```python
from build123d import *

# Parameters (mm, degrees)
SKETCH1_W           = 27.94
SKETCH1_H           = 17.78
SKETCH1_W_2         = 2.54
SKETCH1_H_2         = 12.7
BOSS_EXTRUDE2_DEPTH = 2.54
SKETCH3_R           = 1.27
BOSS_EXTRUDE3_DEPTH = 3.302
SKETCH6_W           = 2.503557337
SKETCH6_H           = 12.554229347
BOSS_EXTRUDE6_DEPTH = 3.302
SKETCH4_W           = 27.94
SKETCH4_H           = 17.78
SKETCH4_W_2         = 2.54
SKETCH4_H_2         = 12.7
BOSS_EXTRUDE7_DEPTH = 2.54


with BuildPart() as part:
    # Sketch1 → Boss-Extrude2 (new body)
    with BuildSketch(Plane(origin=(0, 0, 0), x_dir=(1, 0, 0), z_dir=(0, 1, 0))):
        Rectangle(SKETCH1_W, SKETCH1_H)
        with Locations((-10.20489899, 0)):
            Rectangle(SKETCH1_W_2, SKETCH1_H_2, mode=Mode.SUBTRACT)
        with Locations((10.20489899, 0)):
            Rectangle(SKETCH1_W_2, SKETCH1_H_2, mode=Mode.SUBTRACT)
    extrude(amount=BOSS_EXTRUDE2_DEPTH)

    # Sketch3 → Boss-Extrude3 (add)
    with BuildSketch(Plane(origin=(0, 2.54, 0), x_dir=(1, 0, 0), z_dir=(0, 1, 0))):
        with Locations(Location((-5.318941048, 2.54, 0), (0, 0, 90))):
            Circle(SKETCH3_R)
        with Locations(Location((5.318941048, 2.54, 0), (0, 0, 90))):
            Circle(SKETCH3_R)
    extrude(amount=BOSS_EXTRUDE3_DEPTH)

    # Sketch6 → Boss-Extrude6 (add)
    with BuildSketch(Plane(origin=(0, 2.54, 0), x_dir=(1, 0, 0), z_dir=(0, 1, 0))):
        Polygon((-7.215647318, 4.760339872), (7.384221332, 4.760339872), (7.384221332, -8.817114674), (13.988221332, -8.817114674), (13.97, 8.89), (-13.97, 8.89), (-13.97, -8.89), (-7.347778668, -8.89), align=None)
        with Locations((10.223120322, 0.072885327)):
            Rectangle(SKETCH6_W, SKETCH6_H, mode=Mode.SUBTRACT)
        with Locations((-10.186677659, 0.072885327)):
            Rectangle(SKETCH6_W, SKETCH6_H, mode=Mode.SUBTRACT)
    extrude(amount=BOSS_EXTRUDE6_DEPTH)

    # Sketch4 → Boss-Extrude7 (add)
    with BuildSketch(Plane(origin=(0, 5.842, 0), x_dir=(1, 0, 0), z_dir=(0, 1, 0))):
        with Locations((0.018221332, 0.072885326)):
            Rectangle(SKETCH4_W, SKETCH4_H)
        with Locations((-10.186677658, 0.072885326)):
            Rectangle(SKETCH4_W_2, SKETCH4_H_2, mode=Mode.SUBTRACT)
        with Locations((10.223120322, 0.072885326)):
            Rectangle(SKETCH4_W_2, SKETCH4_H_2, mode=Mode.SUBTRACT)
    extrude(amount=BOSS_EXTRUDE7_DEPTH)


solid = part.part
```
Geometry: final body of the model. Coordinates: model frame, mm. A direction names the side the tool comes from. Round coordinates to 2 decimals unless told otherwise and drop trailing zeros. Loops run counter-clockwise (first coordinate to the right, second up) from the corner with the lowest first, then second, coordinate; pieces in that order, holes last.
Item 1: Section D-D, the plane y = 1.25. Output: boundary loops of the cut face in (x, z).
Checked values:
outline: (-13.97, -8.89) - (13.97, -8.89) - (13.97, 8.89) - (-13.97, 8.89) - close; hole (-11.47, -6.35) - (-8.93, -6.35) - (-8.93, 6.35) - (-11.47, 6.35) - close; hole (8.93, -6.35) - (11.47, -6.35) - (11.47, 6.35) - (8.93, 6.35) - close
Item 2: Contact query for flat-ended pins moving along their axis: P1, Ø1.7, axis at y = 4, z = 1, coming from the +X side; P2, Ø2, axis at x = 10.5, y = 3.5, coming from the -Z side; P3, Ø3, axis at x = -10.5, z = -1, coming from the +Y side; P4, Ø5, axis at x = -2.5, y = 6.5, coming from the +Z side. Output: stop coordinate, or through.
Checked values:
P1: stops at x = 13.98
P2: stops at z = -8.89
P3: stops at y = 8.38
P4: stops at z = 8.82
Item 3: Reachability of faces 1 (the flat face through (3, 7, 8.817)), 2 (the flat face through (-13.97, 3, 0)), 3 (the flat face through (10, 7, -6.423)), 4 (the flat face through (10, 1, 6.35)) from +Z, -Z, +X, -X, +Y, -Y: full face, straight path, thin tool, end or side. Return the list, or none.
Checked values:
face 1: +Z, +X, +Y
face 2: +Z, -Z, -X, +Y, -Y
face 3: +Y
face 4: -Y
Item 4: Section C-C, the plane z = 5. State how many separate pieces and enclosed holes the cut face has, plus the area to 3 significant figures.
Checked values:
separate pieces: 3
enclosed holes: 1
area: 143 mm2
Item 5: Section A-A, the plane x = -10.5. Output: boundary loops of the cut face in (y, z), plus the area to 3 significant figures.
Checked values:
outline: (0, -8.89) - (5.84, -8.89) - (5.84, -8.96) - (8.38, -8.96) - (8.38, -6.42) - (5.84, -6.42) - (5.84, -6.35) - (0, -6.35) - close; (0, 6.35) - (2.54, 6.35) - (2.54, 6.2) - (5.84, 6.2) - (5.84, 6.28) - (8.38, 6.28) - (8.38, 8.82) - (5.84, 8.82) - (5.84, 8.89) - (0, 8.89) - close
area: 43.1 mm2
Item 6: Mould query, pull axis X, two halves, no side actions, for faces 5 (the flat face through (-11.475, 1, 0)), 6 (the flat face through (-13.952, 7, 0)), 7 (the flat face through (13.97, 1, 0)). Classes: released by +X, released by -X, zero draft, split by the parting line, or undercut.
Checked values:
face 5: undercut
face 6: released by -X
face 7: released by +X
Item 7: Section B-B, the plane y = 3.5. Output: boundary loops of the cut face in (x, z).
Checked values:
outline: (-13.97, -8.89) - (13.97, -8.89) - (13.99, 8.82) - (7.38, 8.82) - (7.38, -4.76) - (-7.22, -4.76) - (-7.35, 8.89) - (-13.97, 8.89) - close; circle Ø2.54 at (-5.32, -2.54); circle Ø2.54 at (5.32, -2.54); hole (-11.44, -6.35) - (-8.93, -6.35) - (-8.93, 6.2) - (-11.44, 6.2) - close; hole (8.97, -6.35) - (11.47, -6.35) - (11.47, 6.2) - (8.97, 6.2) - close
Item 8: Line query: L1, parallel to X at y = 6, z = 5.5; L2, parallel to X at y = 2.5, z = 3.5; L3, parallel to Z at x = 10.5, y = 5. Output: solid intervals per line, ascending.
Checked values:
L1: x = -13.95 to -11.46, -8.92 to 8.95, 11.49 to 13.99
L2: x = -13.97 to -11.47, -8.93 to 8.93, 11.47 to 13.97
L3: z = -8.89 to -6.35, 6.2 to 8.82
